Autodesk Inventor part; units mm, degrees
ref_plane "YZ Plane" through (0, 0, 0) normal (1, 0, 0) x (0, 1, 0)
ref_plane "XZ Plane" through (0, 0, 0) normal (0, 1, 0) x (-1, 0, 0)
ref_plane "XY Plane" through (0, 0, 0) normal (0, 0, 1) x (1, 0, 0)
sketch "Sketch1" plane through (0, 0, 0) normal (0, 1, 0) x (-1, 0, 0)
  line L0 (155, -70) -> (155, -210)
  line L1 (155, -210) -> (5, -210)
  line L2 (5, -210) -> (5, -70)
  line L3 (50, -210) -> (110, -210)
  line L4 (5, -70) -> (155, -70)
  line L5 (5, -70) -> (55, -70)
  line L6 (155, -150) -> (135, -150)
  line L7 (135, -150) -> (135, -130)
  line L8 (135, -130) -> (155, -130)
  line L9 (155, -130) -> (155, -150)
  line L10 (5, -150) -> (25, -150)
  line L11 (25, -150) -> (25, -130)
  line L12 (25, -130) -> (5, -130)
  line L13 (5, -180) -> (155, -180) construction
  line L14 (50, -180) -> (110, -180)
  line L15 (110, -180) -> (110, -210)
  line L16 (110, -210) -> (50, -210)
  line L17 (50, -210) -> (50, -180)
  line L18 (110, -210) -> (50, -210)
  line L19 (155, -180) -> (110, -180)
  line L20 (50, -180) -> (5, -180)
  line L21 (135, -30) -> (155, -30)
  line L22 (160, -70) -> (0, -70)
  line L23 (0, -70) -> (0, 0)
  line L24 (0, 0) -> (160, 0)
  line L25 (160, 0) -> (160, -70)
  line L26 (80, -210) -> (80, 0) construction
  line L27 (0, -70) -> (50, -70)
  line L28 (50, -70) -> (50, -65)
  line L29 (50, -65) -> (0, -65)
  line L30 (0, -65) -> (0, -70)
  line L31 (155, -70) -> (105, -70)
  line L32 (160, -70) -> (110, -70)
  line L33 (110, -70) -> (110, -65)
  line L34 (110, -65) -> (160, -65)
  line L35 (160, -65) -> (160, -70)
  line L36 (110, 0) -> (50, 0)
  line L37 (50, 0) -> (50, -5)
  line L38 (50, -5) -> (110, -5)
  line L39 (110, -5) -> (110, 0)
  point P0 (5, -100)
  point P1 (5, -120)
  point P2 (160, -65)
  point P3 (155, 0)
  point P4 (135, 0)
  point P5 (0, -65)
  point P6 (50, -70)
  point P7 (110, -70)
  point P8 (50, 0)
  point P9 (50, -70)
  point P10 (110, -70)
  point P11 (155, -70)
  point P12 (5, -70)
  dimension "d10" = 20
  dimension "d11" = 20
  dimension "d18" = 150
  dimension "d19" = 160
  dimension "d20" = 80
  dimension "d21" = 45
  dimension "d22" = 45
  dimension "d23" = 50
  dimension "d24" = 5
  dimension "d25" = 5
  dimension "d26" = 30
  dimension "d27" = 110
  dimension "d28" = 70
  dimension "d29" = 210
  dimension "d30" = 20
extrude "Extrusion1" add sketch "Sketch1" along normal blind 5 contours L0 L8 L7 L6 L19 L14 L20 L2 L10 L11 L12 L4 | L4 L28 L29 L23 L24 L37 L38 L39 L25 L34 L33 | L15 L1 L17 L14
properties part number "HOOD_1" material "Acrylic"
The model under review builds one solid part; all positions refer to its coordinate system, in mm. A direction names the side the tool comes from. Round coordinates to 2 decimals unless told otherwise and drop trailing zeros. Loops run counter-clockwise (first coordinate to the right, second up) from the corner with the lowest first, then second, coordinate; pieces in that order, holes last. Notation, with made-up numbers: (38, 60.25) -> (74, 60.25) arc R11 cw to (74, 70.25) -> close; hole circle Ø2 at (50, -31). An arc over 180 degrees is marked (long way). One line per question, with ' | ' between items. Start each with the question number.
Item 1: For pin 1 (2.5 mm diameter, centred on y = 3.5, z = -165.5, fed in from +X); pin 2 (2.5 mm diameter, centred on y = 3, z = -66.5, fed in from -X); pin 3 (2.5 mm diameter, centred on y = 2, z = -108.5, fed in from -X), all flat-tipped, find the tip position at first contact; note any pin that passes through.
Item 2: Wall thickness on line 1 along Z through (x, y) = (-117.5, 1.4); line 2 along Z through (x, y) = (-102, 4.65); line 3 along X through (y, z) = (1.6, -122): over which ranges is each line inside the solid? List them lowest first. Write a range as [from, to].
Item 3: Add section D-D, the plane z = -143. Write out the cut boundary in (x, y), then the cut area to 3 significant figures.
Item 4: Add section B-B, the plane x = -21.5. Write out the cut boundary in (y, z), then the cut area to 3 significant figures.
Item 5: Add section A-A, the plane x = -129.5. Write out the cut boundary in (y, z), then the cut area to 3 significant figures.
Item 6: Machinability: for faces 1 (the face through (-110, 2, -195)), 2 (the face through (-5, 2, -100)), 3 (the face through (-25, 2, -140)), 4 (the face through (-135, 2, -65)), which of the approach directions +Z, -Z, +X, -X, +Y, -Y give a long, thin tool a straight path to every point of the face, cutting with its end or side? Answer none if there is none.
Item 7: Add section C-C, the plane y = 1.2. Write out the cut boundary in (x, z), then the cut area to 3 significant figures.
Item 8: Draft analysis for pull direction Z (two halves, no side actions). For faces 5 (the face through (0, 2, -33)), 6 (the face through (-135, 2, 0)), 7 (the face through (-25, 2, -65)), state which applies: +Z half, -Z half, draft (parallel to the pull), parting line (faces both ways), or undercut.
Return value:
1) pin 1: stops at x = -5 | pin 2: stops at x = -110 | pin 3: stops at x = -155
2) line 1: z = [-180, -70], [-65, 0] | line 2: z = [-210, -5] | line 3: x = [-155, -5]
3) outline: (-135, 0) -> (-25, 0) -> (-25, 5) -> (-135, 5) -> close | area: 550 mm2
4) outline: (0, -180) -> (5, -180) -> (5, -150) -> (0, -150) -> close; (0, -130) -> (5, -130) -> (5, -70) -> (0, -70) -> close; (0, -65) -> (5, -65) -> (5, 0) -> (0, 0) -> close | area: 775 mm2
5) outline: (0, -180) -> (5, -180) -> (5, -70) -> (0, -70) -> close; (0, -65) -> (5, -65) -> (5, 0) -> (0, 0) -> close | area: 875 mm2
6) face 1: -Z, -X, +Y, -Y | face 2: -Z, +X, +Y, -Y | face 3: +X, +Y, -Y | face 4: -X, +Y, -Y
7) outline: (-160, -65) -> (-110, -65) -> (-110, -70) -> (-155, -70) -> (-155, -130) -> (-135, -130) -> (-135, -150) -> (-155, -150) -> (-155, -180) -> (-110, -180) -> (-110, -210) -> (-50, -210) -> (-50, -180) -> (-5, -180) -> (-5, -150) -> (-25, -150) -> (-25, -130) -> (-5, -130) -> (-5, -70) -> (-50, -70) -> (-50, -65) -> (0, -65) -> (0, 0) -> (-50, 0) -> (-50, -5) -> (-110, -5) -> (-110, 0) -> (-160, 0) -> close | area: 27,900 mm2
8) face 5: draft | face 6: +Z half | face 7: undercut
